from build123d import *

# Parameters (mm, degrees)
SKETCH1_R           = 377.5
SKETCH1_R_2         = 13
BOSS_EXTRUDE1_DEPTH = 12.5


with BuildPart() as part:
    # Sketch1 → Boss-Extrude1 (new, symmetric)
    with BuildSketch(Plane(origin=(0, 0, 0), x_dir=(1, 0, 0), z_dir=(0, 1, 0))):
        with Locations(Location((0, 0, 0), (0, 0, 270))):
            Circle(SKETCH1_R)
        with Locations(Location((0, 352.5, 0), (0, 0, 270))):
            Circle(SKETCH1_R_2, mode=Mode.SUBTRACT)
        with Locations(Location((108.928490517, 335.247421994, 0), (0, 0, 270))):
            Circle(SKETCH1_R_2, mode=Mode.SUBTRACT)
        with Locations(Location((207.194301433, 285.178490517, 0), (0, 0, 270))):
            Circle(SKETCH1_R_2, mode=Mode.SUBTRACT)
        with Locations(Location((285.178490517, 207.194301433, 0), (0, 0, 270))):
            Circle(SKETCH1_R_2, mode=Mode.SUBTRACT)
        with Locations(Location((335.247421994, 108.928490517, 0), (0, 0, 270))):
            Circle(SKETCH1_R_2, mode=Mode.SUBTRACT)
        with Locations(Location((352.5, 0, 0), (0, 0, 270))):
            Circle(SKETCH1_R_2, mode=Mode.SUBTRACT)
        with Locations(Location((335.247421994, -108.928490517, 0), (0, 0, 270))):
            Circle(SKETCH1_R_2, mode=Mode.SUBTRACT)
        with Locations(Location((285.178490517, -207.194301433, 0), (0, 0, 270))):
            Circle(SKETCH1_R_2, mode=Mode.SUBTRACT)
        with Locations(Location((207.194301433, -285.178490517, 0), (0, 0, 270))):
            Circle(SKETCH1_R_2, mode=Mode.SUBTRACT)
        with Locations(Location((108.928490517, -335.247421994, 0), (0, 0, 270))):
            Circle(SKETCH1_R_2, mode=Mode.SUBTRACT)
        with Locations(Location((0, -352.5, 0), (0, 0, 270))):
            Circle(SKETCH1_R_2, mode=Mode.SUBTRACT)
        with Locations(Location((-108.928490517, -335.247421994, 0), (0, 0, 270))):
            Circle(SKETCH1_R_2, mode=Mode.SUBTRACT)
        with Locations(Location((-207.194301433, -285.178490517, 0), (0, 0, 270))):
            Circle(SKETCH1_R_2, mode=Mode.SUBTRACT)
        with Locations(Location((-285.178490517, -207.194301433, 0), (0, 0, 270))):
            Circle(SKETCH1_R_2, mode=Mode.SUBTRACT)
        with Locations(Location((-335.247421994, -108.928490517, 0), (0, 0, 270))):
            Circle(SKETCH1_R_2, mode=Mode.SUBTRACT)
        with Locations(Location((-352.5, 0, 0), (0, 0, 270))):
            Circle(SKETCH1_R_2, mode=Mode.SUBTRACT)
        with Locations(Location((-335.247421994, 108.928490517, 0), (0, 0, 270))):
            Circle(SKETCH1_R_2, mode=Mode.SUBTRACT)
        with Locations(Location((-285.178490517, 207.194301433, 0), (0, 0, 270))):
            Circle(SKETCH1_R_2, mode=Mode.SUBTRACT)
        with Locations(Location((-207.194301433, 285.178490517, 0), (0, 0, 270))):
            Circle(SKETCH1_R_2, mode=Mode.SUBTRACT)
        with Locations(Location((-108.928490517, 335.247421994, 0), (0, 0, 270))):
            Circle(SKETCH1_R_2, mode=Mode.SUBTRACT)
    extrude(amount=BOSS_EXTRUDE1_DEPTH, both=True)


solid = part.part
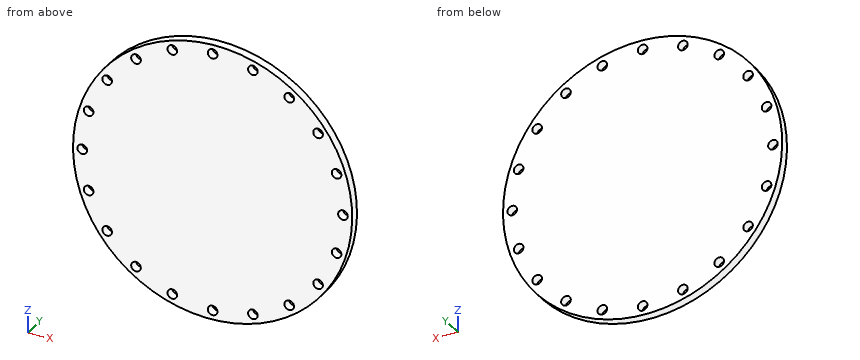
For this review, take the finished solid that the model builds, in its own axes (mm). Round coordinates to 2 decimals unless told otherwise and drop trailing zeros. Order: outer loops, then holes, each group sorted by start corner. A loop starts at its lowest first (then second) coordinate and runs counter-clockwise, first axis right, second up. Notation, with made-up numbers: (-37.5, 49.5) -> (9.5, 49.5) arc R25 ccw to (9.5, 85.5) -> close; hole circle Ø2 at (56.25, 56). An arc over 180 degrees is marked (long way). Put each result on its own line as item: value.
Q1. Add section A-A on z = 0. Write out the cut boundary in (x, y), plus the area to 3 significant figures.
Check result:
outline: (-377.5, -12.5) -> (-365.5, -12.5) -> (-365.5, 12.5) -> (-377.5, 12.5) -> close; (-339.5, -12.5) -> (339.5, -12.5) -> (339.5, 12.5) -> (-339.5, 12.5) -> close; (365.5, -12.5) -> (377.5, -12.5) -> (377.5, 12.5) -> (365.5, 12.5) -> close
area: 17,600 mm2
Q2. Add section C-C on y = 2.5. State how many separate pieces and enclosed holes the cut face has, plus the area to 3 significant figures.
Check result:
separate pieces: 1
enclosed holes: 20
area: 437,000 mm2
Q3. Add section B-B on x = 0. Write out the cut boundary in (y, z).
Check result:
outline: (-12.5, -377.5) -> (12.5, -377.5) -> (12.5, -365.5) -> (-12.5, -365.5) -> close; (-12.5, -339.5) -> (12.5, -339.5) -> (12.5, 339.5) -> (-12.5, 339.5) -> close; (-12.5, 365.5) -> (12.5, 365.5) -> (12.5, 377.5) -> (-12.5, 377.5) -> close
Q4. Insertion check: pin 1 Ø15.5 at (x, z) = (-108.93, 335.25) entering from -Y; pin 2 Ø1.5 at (x, y) = (-40, -8) entering from -Z; pin 3 Ø1 at (x, y) = (-281.5, 5.5) entering from -Z; pin 4 Ø1.5 at (x, y) = (-80.5, 2) entering from -Z. Each pin has a flat end and moves straight along its axis. Give the tip position at first contact, or say it passes through.
Check result:
pin 1: through
pin 2: z = -375.45
pin 3: z = -252.08
pin 4: z = -368.98
Q5. Add section D-D on x = 80.5. Write out the cut boundary in (y, z).
Check result:
outline: (-12.5, -368.82) -> (12.5, -368.82) -> (12.5, 368.82) -> (-12.5, 368.82) -> close
Q6. For probe 1 along X at (y, z) = (-5.5, 205); probe 2 along Z at (x, y) = (-2, 4.5); probe 3 along X at (y, z) = (3.5, -199), list the stretches that pass through material, from the lowest coordinate up. Write a range as [from, to].
Check result:
probe 1: [-316.99, -297.99], [-272.37, 272.37], [297.99, 316.99]
probe 2: [-377.49, -365.35], [-339.65, 339.65], [365.35, 377.49]
probe 3: [-320.79, -295.27], [-275.09, 275.09], [295.27, 320.79]
